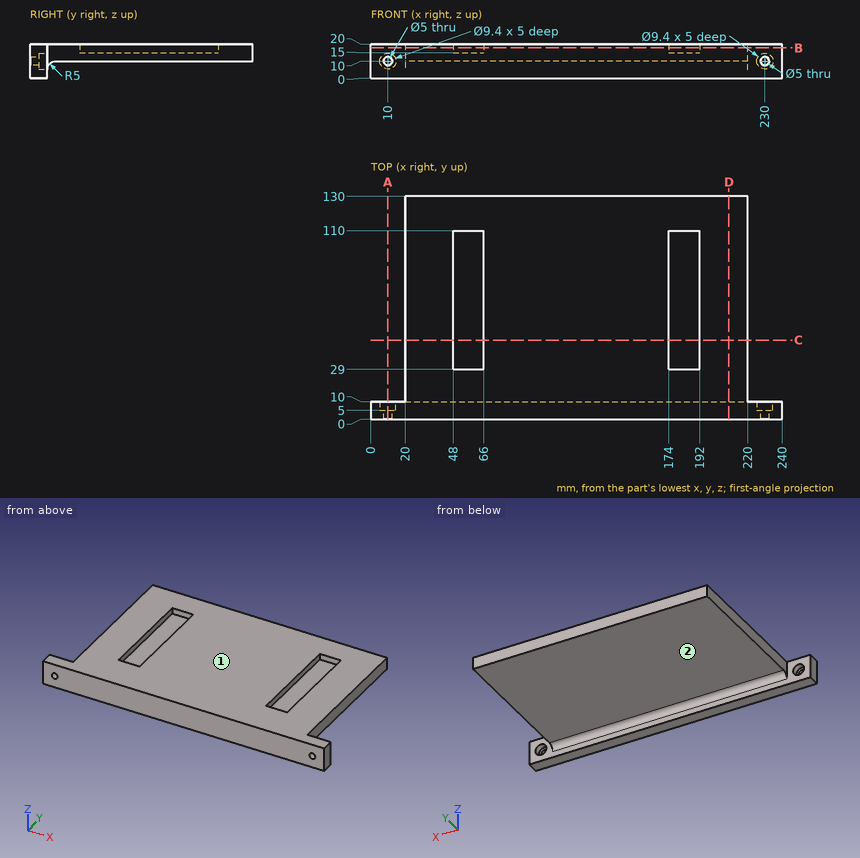
For this review, use the dimensioned drawing (mm, ordinates from the lowest corner) and the shaded views. A direction names the side the tool comes from. Coordinates: 2 decimals unless noted, no trailing zeros. Write each loop counter-clockwise with the first axis right and the second up, starting at its lowest first coordinate (ties: lowest second). Pieces come first, ordered by that corner, then holes. Notation, with made-up numbers: (87, 70) - (137, 70) arc R6 ccw to (137, 81) - close; hole circle Ø3 at (62, -26.75). An arc over 180 degrees is marked (long way). Answer in a Markdown table with one row per item. Add a question column.
Q1. Consider section B-B on z = 17.75. Give the boundary of the cut face in (x, y), then the cut area to 3 significant figures.
Q2. Consider section A-A on x = 10. Give the boundary of the cut face in (y, z).
Q3. For the marked faces 1 and 2, list the 3-axis set-ups (+Z, -Z, +X, -X, +Y, -Y) from which the entire face can be reached by the end or side of a thin tool; tool diameter is ignored.
Q4. Clearance check with flat-ended pins moving along their axes: pin 1 (5.5 mm diameter, centred on x = 230, z = 10, fed in from +Y); pin 2 (7.5 mm diameter, centred on x = 10, z = 11, fed in from +Y); pin 3 (4 mm diameter, centred on y = 76.5, z = 18, fed in from -X). State where each tip first meets the part, or that it passes through.
Q5. To check wall thickness, follow line 1 along X through (y, z) = (37.5, 17.5); line 2 along Z through (x, y) = (230, 8.6); line 3 along Y through (x, z) = (185, 18.5). State the ranges of each line that lie inside material, in increasing order. Write a range as from..to.
Q6. Consider section C-C on y = 46. Give the boundary of the cut face in (x, z), then the cut area to 3 significant figures.
Q7. Consider section D-D on x = 209. Give the boundary of the cut face in (y, z).
Answers below:
| question | item | result |
|---|---|---|
| 1 | outline | (0, 0) - (240, 0) - (240, 10) - (220, 10) - (220, 130) - (20, 130) - (20, 10) - (0, 10) - close; hole (48, 29) - (66, 29) - (66, 110) - (48, 110) - close; hole (174, 29) - (192, 29) - (192, 110) - (174, 110) - close |
| 1 | area | 23,500 mm² |
| 2 | outline | (0, 0) - (10, 0) - (10, 5.3) - (5, 5.3) - (5, 7.5) - (0, 7.5) - close; (0, 12.5) - (5, 12.5) - (5, 14.7) - (10, 14.7) - (10, 20) - (0, 20) - close |
| 3 | face 1 | +Z, +X, -X, +Y, -Y |
| 3 | face 2 | -Z, +X, -X, +Y |
| 4 | pin 1 | y = 5 |
| 4 | pin 2 | y = 10 |
| 4 | pin 3 | x = 20 |
| 5 | line 1 | 20..48, 66..174, 192..220 |
| 5 | line 2 | 0..5.3, 14.7..20 |
| 5 | line 3 | 0..29, 110..130 |
| 6 | outline | (20, 10) - (220, 10) - (220, 20) - (192, 20) - (192, 15) - (174, 15) - (174, 20) - (66, 20) - (66, 15) - (48, 15) - (48, 20) - (20, 20) - close |
| 6 | area | 1,820 mm² |
| 7 | outline | (0, 0) - (10, 0) - (10, 5) arc R5 cw to (15, 10) - (130, 10) - (130, 20) - (0, 20) - close |
